Input: dimensioned drawing with shaded views. Units: mm. Origin: part minimum x, y, z. Round coordinates to 2 decimals unless told otherwise and drop trailing zeros. Order: outer loops, then holes, each group sorted by start corner. A loop starts at its lowest first (then second) coordinate and runs counter-clockwise, first axis right, second up. Notation, with made-up numbers: (-11.5, 74.5) - (35.5, 74.5) arc R25 ccw to (35.5, 111.5) - close; hole circle Ø9 at (-3, -35). An arc over 180 degrees is marked (long way). Put each result on its own line as item: value. Start each with the question number.
(1) Material intervals for L1, parallel to X at y = 1.25, z = 50.8; L2, parallel to Z at x = 215.9, y = 2.45; L3, parallel to X at y = 1.4, z = 50, sorted ascending. Write a range as [from, to].
(2) Section B-B (z = 50.8). Output: boundary loops of the cut face in (x, y) (3 decimals).
(3) Section A-A (x = 215.9). Output: boundary loops of the cut face in (y, z) (3 decimals), and give its area (3 significant figures).
(4) Pin query (flat end, axial travel): P1, Ø8, axis at x = 215.9, z = 50.8, coming from the +Y side (3 decimals); P2, Ø5.5, axis at x = 12.7, z = 50.8, coming from the -Y side. Return the tip coordinate at first contact, or that it passes through.
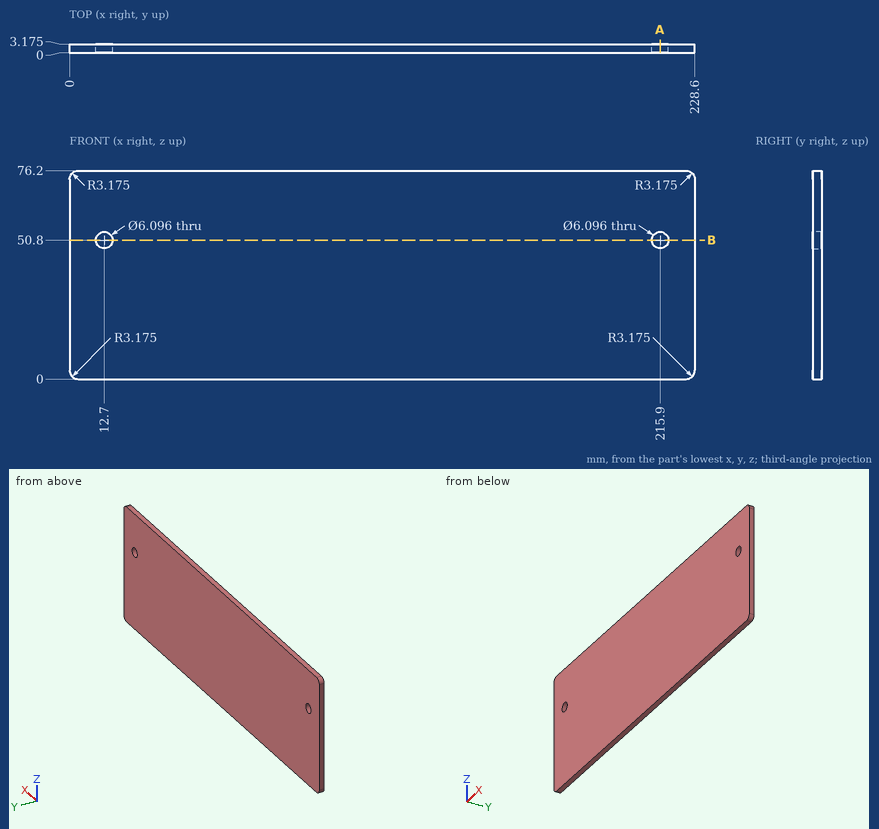
Checks:
1. L1: x = [0, 9.65], [15.75, 212.85], [218.95, 228.6]
1. L2: z = [0, 47.75], [53.85, 76.2]
1. L3: x = [0, 9.76], [15.64, 212.96], [218.84, 228.6]
2. outline: (0, 0) - (9.652, 0) - (9.652, 3.175) - (0, 3.175) - close; (15.748, 0) - (212.852, 0) - (212.852, 3.175) - (15.748, 3.175) - close; (218.948, 0) - (228.6, 0) - (228.6, 3.175) - (218.948, 3.175) - close
3. outline: (0, 0) - (3.175, 0) - (3.175, 47.752) - (0, 47.752) - close; (0, 53.848) - (3.175, 53.848) - (3.175, 76.2) - (0, 76.2) - close
3. area: 223 mm²
4. P1: stops at y = 3.175
4. P2: passes through
